Part model, mm, in its own coordinate system. A direction names the side the tool comes from. Give positions to 0.01 mm unless a question says otherwise; leave off trailing zeros. Write each loop counter-clockwise with the first axis right and the second up, starting at its lowest first coordinate (ties: lowest second). Pieces come first, ordered by that corner, then holes.
Autodesk Inventor part; units mm, degrees
ref_plane "YZ Plane" through (0, 0, 0) normal (1, 0, 0) x (0, 1, 0)
ref_plane "XZ Plane" through (0, 0, 0) normal (0, 1, 0) x (-1, 0, 0)
ref_plane "XY Plane" through (0, 0, 0) normal (0, 0, 1) x (1, 0, 0)
sketch "Sketch1" plane through (0, 0, 0) normal (0, 0, 1) x (1, 0, 0)
  line L0 (-152.4, 6.35) -> (152.4, 6.35)
  line L1 (152.4, 6.35) -> (152.4, -6.35)
  line L2 (152.4, -6.35) -> (-152.4, -6.35)
  line L3 (-152.4, -6.35) -> (-152.4, 6.35)
  line L4 (-152.4, 6.35) -> (152.4, -6.35) construction
  line L5 (152.4, 6.35) -> (-152.4, -6.35) construction
  line L6 (-152.4, 0) -> (-146.05, 0)
  line L7 (-152.4, -31.75) -> (-139.7, -31.75)
  line L8 (-139.7, -31.75) -> (-139.7, 31.75)
  line L9 (-139.7, 31.75) -> (-152.4, 31.75)
  line L10 (-152.4, 31.75) -> (-152.4, -31.75)
  line L11 (-152.4, -31.75) -> (-139.7, 31.75) construction
  line L12 (-139.7, -31.75) -> (-152.4, 31.75) construction
  line L13 (-152.4, 0) -> (-165.1, 0)
  line L14 (-165.1, 0) -> (-152.4, 6.35)
  line L15 (152.4, 0) -> (152.4, 44.45)
  line L16 (152.4, 44.45) -> (113.1983, 0)
  line L17 (-146.05, 0) -> (152.4, 0)
  line L18 (152.4, 0) -> (152.4, -44.45)
  line L19 (152.4, -44.45) -> (113.1983, 0)
  point P0 (0, 0)
  point P1 (-139.7, 6.35)
  dimension "d0" = 304.8
  dimension "d1" = 12.7
  dimension "d2" = 6.35
  dimension "d3" = 12.7
  dimension "d4" = 63.5
  dimension "d5" = 12.7
  dimension "d6" = 44.45
  dimension "d8" = 41.41
revolve "Revolution1" add sketch "Sketch1" angle 360 about axis through (-146.05, 0, 0) along (1, 0, 0) contours L10 L9 L8 L0 | L0 L8 L17 L6 L3 | L3 L13 L14 | L0 L16 L17 L8 | L0 L1 L17 L16
extrude "Extrusion1" add sketch "Sketch1" along normal mid plane 6.35 contours L16 L15 L0 | L0 L1 L17 L16 | L17 L1 L2 L19 | L2 L18 L19
sketch "Sketch2" plane through (-139.7, 0, 0) normal (1, 0, 0) x (0, 0, -1)
  circle A0 centre (0, 0) radius 63.5
  circle A1 centre (0, 0) radius 6.35
  line L0 (0, 0) -> (0, 63.5)
  line L1 (0, 0) -> (54.9926, -31.75)
  line L2 (0, 0) -> (-54.9926, -31.75)
  line L3 (0, 0) -> (54.9926, 31.75)
  line L4 (0, 0) -> (0, -63.5)
  line L5 (0, 0) -> (-54.9926, 31.75)
  circle A2 centre (0, 0) radius 31.75
  point P0 (0, -31.75)
  point P1 (-27.4963, -15.875)
  point P2 (27.4963, 15.875)
  point P3 (27.4963, -15.875)
  point P4 (-27.4963, 15.875)
  point P5 (0, 31.75)
  dimension "d12" = 12.7
  dimension "d13" = 120
  dimension "d14" = 120
  dimension "d15" = 60
  dimension "d16" = 60
extrude "Extrusion2" add sketch "Sketch2" against normal blind 12.7 contours A0 L1 A2 L3 | L0 A2 L5 A0 | A0 L2 A2 L4
properties part number "Powder Arrow"
1) Two-plate mould, pull along Z, no slides. Class faces 5 (the face through (-145.96, 23.7, -41.05)), 6 (the face through (135.465, -25.247, -0.044)), 7 (the face through (143, 17, 3.175)): +Z half, -Z half, draft (parallel to the pull), parting line (faces both ways), or undercut.
Answers follow:
face 5: undercut
face 6: draft
face 7: +Z half
2) Pin check, flat tips, straight feed: pin 1 Ø4 at (x, y) = (-148, -51) entering from -Z; pin 2 Ø8 at (x, y) = (72, 1.5) entering from +Z; pin 3 Ø12 at (y, z) = (-13, -47) entering from -X. Stop position of each tip, or through.
Answers follow:
pin 1: stops at z = 0
pin 2: stops at z = 6.35
pin 3: stops at x = -152.4
3) Saw through at A-A, the plane y = 22. Write the cut outline in (x, z) (3 decimals).
Answers follow:
outline: (-152.4, -59.567) - (-139.7, -59.567) - (-139.7, -38.105) - (-152.4, -38.105) - close; (-152.4, -22.892) - (-139.7, -22.892) - (-139.7, 38.105) - (-152.4, 38.105) - close; (132.601, -3.175) - (152.4, -3.175) - (152.4, 3.175) - (132.601, 3.175) - close
4) 3-axis set-ups, long thin cutter, end or side, ignore diameter. For faces 1 (the face through (8.395, -6.344, 0.279)), 2 (the face through (143, -16, -3.175)), 3 (the face through (139, -16, 3.175)), 4 (the face through (143, 17, -3.175)): which of +Z, -Z, +X, -X, +Y, -Y reach the whole face in a straight line?
Answers follow:
face 1: none
face 2: -Z, +X, -Y
face 3: +Z, +X, -Y
face 4: -Z, +X, +Y
5) Saw through at B-B, the plane x = 44. Write the cut outline in (y, z), then the cut area to 3 significant figures.
Answers follow:
outline: circle Ø12.7 at (0, 0)
area: 127 mm2
6) Saw through at D-D, the plane z = -32. Write the cut outline in (x, y), then the cut area to 3 significant figures.
Answers follow:
outline: (-152.4, -18.48) - (-139.7, -18.48) - (-139.7, 18.48) - (-152.4, 18.48) - close
area: 469 mm2
7) Wall check: L1, parallel to X at y = 31.5, z = 36; L2, parallel to X at y = 7.5, z = 2; L3, parallel to Z at x = 43.5, y = -3. Give the ranges that are in metal, low to high.
Answers follow:
L1: x = -152.4 to -139.7
L2: x = -152.4 to -139.7, 119.81 to 152.4
L3: z = -5.6 to 5.6
8) Saw through at C-C, the plane z = -11.5. Write the cut outline in (x, y), then the cut area to 3 significant figures.
Answers follow:
outline: (-152.4, -29.59) - (-139.7, -29.59) - (-139.7, 29.59) - (-152.4, 29.59) - close
area: 752 mm2
